The listing builds one solid part. Answer for the finished solid, in the listing's coordinates (mm). Face numbers are marked on the shaded views. A direction names the side the tool comes from. Coordinates: 2 decimals unless noted, no trailing zeros. Loops run counter-clockwise (first coordinate to the right, second up) from the corner with the lowest first, then second, coordinate; pieces in that order, holes last. Notation, with made-up numbers: M -32.5,66.25 L 19.5,66.25 A35 cw 19.5,98.25 Z; hole C 53.5,-2 d1. An arc over 180 degrees is marked long. Return JSON: item names as keys, results as strings. Group by question number.
1. Section D-D (y = -1) is taken. Write down the section's boundary in (x, z), then the cut area to 3 significant figures.
2. Section C-C (z = 36.5) is taken. Write down the section's boundary in (x, y), then the cut area to 3 significant figures.
3. Section B-B (x = 75) is taken. Write down the section's boundary in (y, z).
4. Which of the six approach directions +Z, -Z, +X, -X, +Y, -Y give full straight-line access (tool end or side, diameter ignored) to the marked faces 5 and 6?
5. Straight lines are drawn through the part: L1, parallel to Y at x = 75, z = -3.5; L2, parallel to X at y = -75, z = -6; L3, parallel to X at y = 4.5, z = -3. For each, find the intervals that lie inside material, in ascending order. Write a range as from..to.
6. Section A-A (y = 75) is taken. Write down the section's boundary in (x, z).
7. Given P1, Ø8, axis at x = 48.5, y = -7, coming from the -Z side; P2, Ø2.5, axis at x = 14, y = 96.5, coming from the -Z side, each flat-ended and moving along its own axis, determine where each tip first touches the part or whether it passes through.
8. The mould has two halves that part along X. Classify the marked faces 1, 2, 3 and 4: pulls with the +X half, pulls with the -X half, needs draft (parallel to the pull), parting line crosses it, or undercut.
Autodesk Inventor part; units mm, degrees
ref_plane "YZ Plane" through (0, 0, 0) normal (1, 0, 0) x (0, 1, 0)
ref_plane "XZ Plane" through (0, 0, 0) normal (0, 1, 0) x (-1, 0, 0)
ref_plane "XY Plane" through (0, 0, 0) normal (0, 0, 1) x (1, 0, 0)
sketch "Sketch3" plane through (0, 0, 0) normal (0, 0, 1) x (1, 0, 0)
  line L0 (-100, -100) -> (100, -100)
  line L1 (100, -100) -> (100, 100)
  line L2 (100, 100) -> (-100, 100)
  line L3 (-100, 100) -> (-100, -100)
  line L4 (-100, -100) -> (100, 100) construction
  line L5 (100, -100) -> (-100, 100) construction
  point P0 (0, 0)
  dimension "d8" = 200
  dimension "d9" = 200
extrude "Extrusion2" add sketch "Sketch3" along normal blind 90
shell "Shell2" thickness 5 removed faces 2 at (-33.3333, -100, 30) at (-33.3333, -33.3333, 0)
sketch "Sketch4" plane through (0, 0, 0) normal (0, 0, 1) x (1, 0, 0)
  line L0 (100, -100) -> (100, 100) construction
  line L1 (100, 100) -> (-100, 100) construction
  line L2 (-100, 100) -> (-100, -100) construction
  line L3 (-100, -100) -> (100, -100) construction
  line L4 (-100, 100) -> (100, 100)
  line L5 (100, 100) -> (100, -100)
  line L6 (-100, -100) -> (-100, 100)
  line L7 (0, -140) -> (0, 140)
  point P0 (0, 0)
  point P1 (-75, -75)
  point P2 (75, -75)
  point P3 (-75, 75)
  point P4 (75, 75)
  dimension "d13" = 150
  dimension "d14" = 25
  dimension "d15" = 150
sketch "Sketch5" plane through (0, 0, 0) normal (0, 0, 1) x (1, 0, 0)
  line L0 (-100, 100) -> (-100, -100)
  line L1 (100, 100) -> (-100, 100)
  line L2 (-100, 100) -> (-100, -100)
  line L3 (100, -100) -> (100, 100)
  line L4 (-100, -100) -> (100, -100)
  line L5 (100, -100) -> (50, -100)
  line L6 (50, -100) -> (50, 100)
  line L7 (-50, -100) -> (-50, 100)
  point P0 (0, 0)
  dimension "d16" = 50
  dimension "d17" = 50
extrude "Extrusion3" add sketch "Sketch5" against normal blind 10 contours L1 L7 L4 L0 | L1 L3 L4 L6
hole "Hole1" at (-75, -75, 0) at (75, -75, 0) at (-75, 75, 0) at (75, 75, 0) direction (0, 0, -1) diameter 5.5 end through all
equation "\"d17\" = d16"
properties part number "KN-00-00-01" material "PET Plastic"
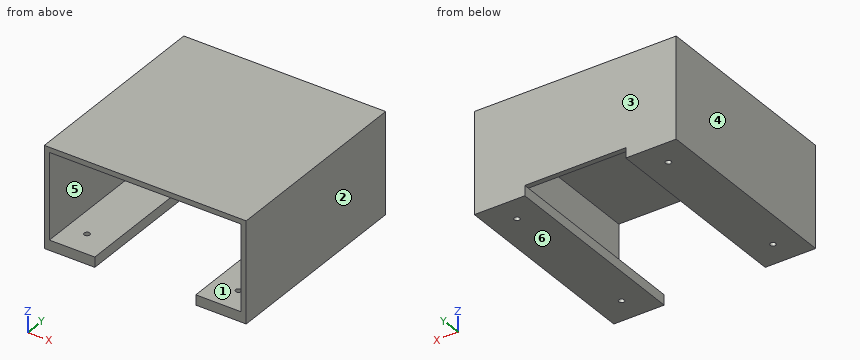
Worked out:
{
 "1": {"outline": "M -100,-10 L -50,-10 L -50,0 L -95,0 L -95,85 L 95,85 L 95,0 L 50,0 L 50,-10 L 100,-10 L 100,90 L -100,90 Z", "area": "2,850 mm^2"},
 "2": {"outline": "M -100,-100 L -95,-100 L -95,95 L 95,95 L 95,-100 L 100,-100 L 100,100 L -100,100 Z", "area": "2,950 mm^2"},
 "3": {"outline": "M -100,-10 L -77.75,-10 L -77.75,0 L -100,0 Z; M -100,85 L 95,85 L 95,0 L 77.75,0 L 77.75,-10 L 100,-10 L 100,90 L -100,90 Z; M -72.25,-10 L 72.25,-10 L 72.25,0 L -72.25,0 Z"},
 "4": {"face 5": "-Y", "face 6": "-Z, +X, -X, +Y, -Y"},
 "5": {"L1": "-100..-77.75, -72.25..72.25, 77.75..100", "L2": "-100..-77.75, -72.25..-50, 50..72.25, 77.75..100", "L3": "-100..-50, 50..100"},
 "6": {"outline": "M -100,-10 L -77.75,-10 L -77.75,0 L -95,0 L -95,85 L 95,85 L 95,0 L 77.75,0 L 77.75,-10 L 100,-10 L 100,90 L -100,90 Z; M -72.25,-10 L -50,-10 L -50,0 L -72.25,0 Z; M 50,-10 L 72.25,-10 L 72.25,0 L 50,0 Z"},
 "7": {"P1": "z = -10", "P2": "z = 0"},
 "8": {"face 1": "undercut", "face 2": "pulls with the +X half", "face 3": "needs draft", "face 4": "pulls with the -X half"}
}
